Part print with two shaded views. Sizes in mm from the minimum x, y, z corner. A direction names the side the tool comes from. Round coordinates to 2 decimals unless told otherwise and drop trailing zeros. Order: outer loops, then holes, each group sorted by start corner. A loop starts at its lowest first (then second) coordinate and runs counter-clockwise, first axis right, second up. Notation, with made-up numbers: M -30,1 L 12,1 A21 cw 12,39 Z; hole C -35.5,66.25 d1. An arc over 180 degrees is marked long. Put each result on its own line as item: value.
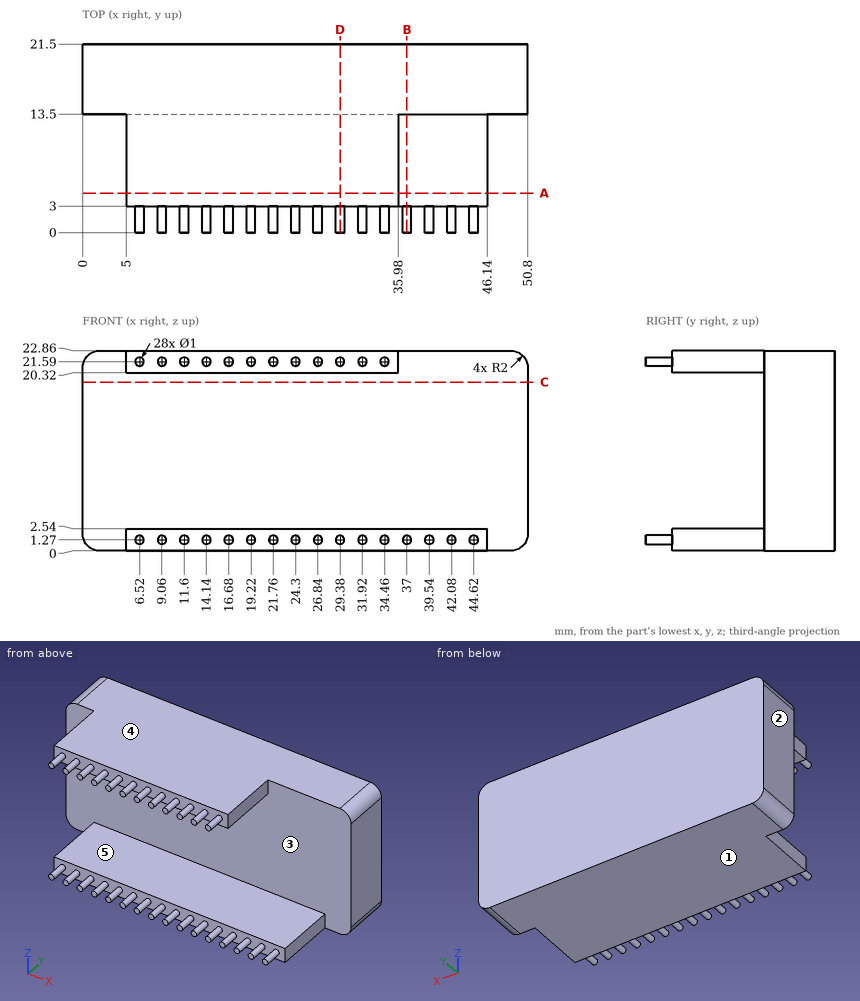
Item 1: Pin check, flat tips, straight feed: P1, Ø3, axis at x = 21, z = 13.5, coming from the -Y side; P2, Ø2, axis at y = 10, z = 21.5, coming from the -X side; P3, Ø3, axis at y = 6.5, z = 1.5, coming from the +X side. Stop position of each tip, or through.
Answers below:
P1: y = 13.5
P2: x = 5
P3: x = 46.14
Item 2: Mould opens along Z. For the marked faces 1, 2 and 3 say: pulls with the +Z half, pulls with the -Z half, needs draft (parallel to the pull), parting line crosses it, or undercut.
Answers below:
face 1: pulls with the -Z half
face 2: needs draft
face 3: undercut
Item 3: Band-saw the part on C-C on z = 19.25. Give the cut face in (x, y), and give its area (3 significant figures).
Answers below:
outline: M 0,13.5 L 50.8,13.5 L 50.8,21.5 L 0,21.5 Z
area: 406 mm²
Item 4: Band-saw the part on A-A on y = 4.5. Give the cut face in (x, z).
Answers below:
outline: M 5,0 L 46.14,0 L 46.14,2.54 L 5,2.54 Z; M 5,20.32 L 35.98,20.32 L 35.98,22.86 L 5,22.86 Z
Item 5: Band-saw the part on B-B on x = 37. Give the cut face in (y, z), and give its area (3 significant figures).
Answers below:
outline: M 0,0.77 L 3,0.77 L 3,0 L 21.5,0 L 21.5,22.86 L 13.5,22.86 L 13.5,2.54 L 3,2.54 L 3,1.77 L 0,1.77 Z
area: 213 mm²
Item 6: Probe line 1 along Z through (x, y) = (35.5, 11.5); line 2 along Y through (x, z) = (21, 16.75); line 3 along Z through (x, y) = (24, 2.75). List the from-to ranges inside material, lowest first. Write a range as [from, to].
Answers below:
line 1: [0, 2.54], [20.32, 22.86]
line 2: [13.5, 21.5]
line 3: [0.87, 1.67], [21.19, 21.99]
Item 7: Tool access for the marked faces 4 and 5: list every direction of +Z, -Z, +X, -X, +Y, -Y with a clear straight run to the whole face (end or side of a thin tool).
Answers below:
face 4: +Z, +X, -X, +Y, -Y
face 5: +X, -X, -Y
Item 8: Band-saw the part on D-D on x = 29.38. Give the cut face in (y, z), and give its area (3 significant figures).
Answers below:
outline: M 0,0.77 L 3,0.77 L 3,0 L 21.5,0 L 21.5,22.86 L 3,22.86 L 3,22.09 L 0,22.09 L 0,21.09 L 3,21.09 L 3,20.32 L 13.5,20.32 L 13.5,2.54 L 3,2.54 L 3,1.77 L 0,1.77 Z
area: 242 mm²
